Work out the finished part from the listing and answer in its coordinate system (mm). A direction names the side the tool comes from. Round coordinates to 2 decimals unless told otherwise and drop trailing zeros. Write each loop counter-clockwise with the first axis right and the second up, starting at its lowest first coordinate (ties: lowest second). Pieces come first, ordered by that corner, then holes. Notation, with made-up numbers: (4, -15) - (42, -15) arc R26 cw to (42, 16) - close; hole circle Ø3 at (35, 21). An arc over 180 degrees is marked (long way). Answer as a JSON object with one key per item and string values.
```python
from build123d import *

# Parameters (mm, degrees)
F1_DEPTH = 12.5
F2_T     = -0.9
F3_DEPTH = 21.6


with BuildPart() as f1:
    # F0 (on Front) → F1 (new body, symmetric)
    with BuildSketch(Plane.XZ):
        Polygon((8.3499658552, -0.0238792301), (4.1956629474, 7.2193429363), (-4.1543029077, 7.2432221663), (-8.3499658552, 0.0238792301), (-4.1956629474, -7.2193429363), (4.1543029077, -7.2432221663), align=None)
    extrude(amount=F1_DEPTH, both=True)

    # F2
    f2_openings = [f1.faces().sort_by_distance(p)[0] for p in [
        (0, 12.5, 0),
    ]]
    offset(amount=F2_T, openings=f2_openings)

    # F3 (add): a face of the model
    f3_faces = [f1.faces().sort_by_distance(p)[0] for p in [
        (0, -11.6, 0),
    ]]
    extrude(f3_faces, amount=F3_DEPTH)


solid = f1.part
```
Item 1: A cutting plane is placed at A-A (y = 7.25). Write down the section's boundary in (x, z).
Results found:
{"outline": "(-8.35, 0.02) - (-4.2, -7.22) - (4.15, -7.24) - (8.35, -0.02) - (4.2, 7.22) - (-4.15, 7.24) - close"}
Item 2: A cutting plane is placed at C-C (x = -3). Write down the section's boundary in (y, z), and give its area (3 significant figures).
Results found:
{"outline": "(-12.5, -7.22) - (12.5, -7.22) - (12.5, -6.32) - (10, -6.32) - (10, 6.34) - (12.5, 6.34) - (12.5, 7.24) - (-12.5, 7.24) - close", "area": "330 mm²"}
Item 3: Each of these flat-tipped pins is pushed along its axis until it touches: P1, Ø6, axis at y = 8.5, z = -1, coming from the +X side; P2, Ø6.5, axis at x = -1.5, z = -0.5, coming from the +Y side; P3, Ø3, axis at y = 2.5, z = -5.5, coming from the -X side. Where does it stop, or does it pass through?
Results found:
{"P1": "x = 8.35", "P2": "y = 10", "P3": "x = -6.04"}
Item 4: Consider line 1 along Z through (x, y) = (4, -6.75); line 2 along Y through (x, z) = (-4.75, -2); line 3 along X through (y, z) = (10.5, 5.75). Determine where each line is inside the solid, lowest interval first.
Results found:
{"line 1": "-7.24 to 7.22", "line 2": "-12.5 to 10", "line 3": "-5.02 to -3.98, 4 to 5.04"}
Item 5: Determine the mould class of faces 3 (the flat face through (0, -12.5, 0)), 4 (the flat face through (-6.3, -0.18, -3.55)), 5 (the flat face through (-6.223, -0.175, 3.684)), 6 (the flat face through (-5.518, 11.232, -3.106)) for opening direction Z: pulls with the +Z half, pulls with the -Z half, needs draft (parallel to the pull), parting line crosses it, or undercut.
Results found:
{"face 3": "needs draft", "face 4": "pulls with the -Z half", "face 5": "pulls with the +Z half", "face 6": "undercut"}
Item 6: For faces 1 (the flat face through (6, 12.5, -3)), 2 (the flat face through (5.518, 11.232, 3.106)), determine the directions among +Z, -Z, +X, -X, +Y, -Y from which every point of the face is accessible in a straight line to the end or side of a thin tool.
Results found:
{"face 1": "+Z, -Z, +X, -X, +Y", "face 2": "+Y"}
Item 7: A cutting plane is placed at B-B (z = -5.5). Write down the section's boundary in (x, y), and give its area (3 significant figures).
Results found:
{"outline": "(-5.18, -12.5) - (5.17, -12.5) - (5.17, 12.5) - (4.13, 12.5) - (4.13, 10) - (-4.14, 10) - (-4.14, 12.5) - (-5.18, 12.5) - close", "area": "238 mm²"}
